Input: part model. Units: mm. Frame: model coordinates. Face numbers are marked on the shaded views. A direction names the side the tool comes from. Coordinates: 2 decimals unless noted, no trailing zeros. Write each loop counter-clockwise with the first axis right and the second up, starting at its lowest first coordinate (ties: lowest second). Pieces come first, ordered by that corner, then holes. Notation, with made-up numbers: M -3,64 L 37,64 A18 cw 37,78 Z; hole C 88,-9 d6. An arc over 180 degrees is marked long. Answer as a JSON object with one key per item and string values. Group by question number.
from build123d import *

# Parameters (mm, degrees)
SKETCH1_W           = 27.94
SKETCH1_H           = 25.4
SKETCH1_W_2         = 25.908
SKETCH1_H_2         = 24.13
BOSS_EXTRUDE1_DEPTH = 2.032
SKETCH2_W           = 27.94
SKETCH2_H           = 25.4
BOSS_EXTRUDE2_DEPTH = 2.54
SKETCH3_R           = 13.843
BOSS_EXTRUDE3_DEPTH = 6.35
FILLET1_R           = 2.54


with BuildPart() as part:
    # Sketch1 → Boss-Extrude1 (new body)
    with BuildSketch(Plane(origin=(0, 0, 0), x_dir=(1, 0, 0), z_dir=(0, 1, 0))):
        Rectangle(SKETCH1_W, SKETCH1_H)
        Rectangle(SKETCH1_W_2, SKETCH1_H_2, mode=Mode.SUBTRACT)
    extrude(amount=BOSS_EXTRUDE1_DEPTH)

    # Sketch2 → Boss-Extrude2 (add)
    with BuildSketch(Plane(origin=(0, 0, 0), x_dir=(1, 0, 0), z_dir=(0, 1, 0))):
        Rectangle(SKETCH2_W, SKETCH2_H)
    extrude(amount=-BOSS_EXTRUDE2_DEPTH)

    # Sketch3 → Boss-Extrude3 (add)
    with BuildSketch(Plane.XZ.offset(2.54)):
        Circle(SKETCH3_R)
    extrude(amount=BOSS_EXTRUDE3_DEPTH)

    # Fillet1
    fillet1_edges = [part.edges().sort_by_distance(p)[0] for p in [
        (13.97, -0.254, 12.7),
        (-13.97, -0.254, 12.7),
        (-13.97, -0.254, -12.7),
        (13.97, -0.254, -12.7),
    ]]
    fillet(fillet1_edges, radius=FILLET1_R)


solid = part.part
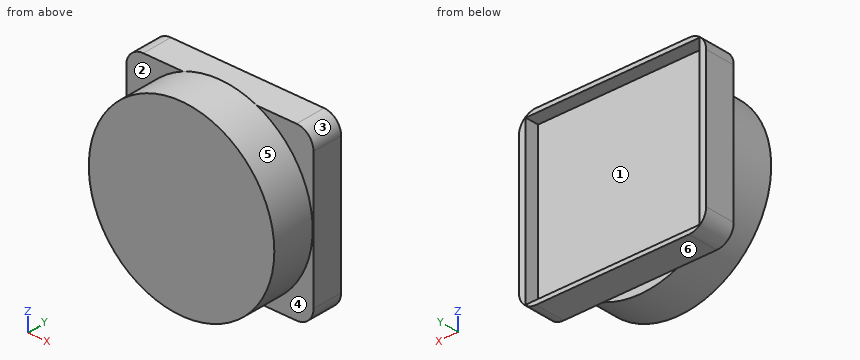
Q1. Access query for the marked faces 4, 5 and 6. Directions: +Z, -Z, +X, -X, +Y, -Y. A direction counts if a zero-diameter tool reaches every point of the face in a straight line with its end or side. Return the directions, or none.
Q2. Draft query along X for the marked faces 1, 2 and 3. Return one class per face: released by +X, released by -X, zero draft, split by the parting line, or undercut.
Q3. Pin query (flat end, axial travel): pin 1 Ø10 at (x, z) = (1.5, 6.5) entering from +Y; pin 2 Ø2.5 at (x, y) = (-2, -1) entering from +Z; pin 3 Ø0.6 at (x, y) = (4, 1.5) entering from -Z. Return the tip coordinate at first contact, or that it passes through.
Q4. Section C-C, the plane x = 0. Return the cut outline in (y, z) (3 decimals), and give its area (3 significant figures).
Q5. Section A-A, the plane y = 0.75. Return the cut outline in (x, z) (3 decimals), and give its area (3 significant figures).
Q6. Section D-D, the plane y = -1.75. Return the cut outline in (x, z).
Q7. Section B-B, the plane z = 0. Return the cut outline in (x, y), and give its area (3 significant figures).
Q8. Line query: line 1 (Z direction, x = -6.75, y = 1) (3 decimals); line 2 (X direction, y = 1.5, z = -5.75); line 3 (Y direction, x = 10.5, z = -1.25). Output: solid intervals per line, ascending. Write a range as from..to.
Filled in:
{
 "1": {"face 4": "+X, -Y", "face 5": "-Y", "face 6": "-Z, +X, -X, +Y"},
 "2": {"face 1": "undercut", "face 2": "zero draft", "face 3": "released by +X"},
 "3": {"pin 1": "y = 0", "pin 2": "z = 12.7", "pin 3": "z = -12.7"},
 "4": {"outline": "M -8.89,-13.843 L -2.54,-13.843 L -2.54,-12.7 L 2.032,-12.7 L 2.032,-12.065 L 0,-12.065 L 0,12.065 L 2.032,12.065 L 2.032,12.7 L -2.54,12.7 L -2.54,13.843 L -8.89,13.843 Z", "area": "243 mm^2"},
 "5": {"outline": "M -13.97,-10.16 A2.54 ccw -11.43,-12.7 L 11.43,-12.7 A2.54 ccw 13.97,-10.16 L 13.97,10.16 A2.54 ccw 11.43,12.7 L -11.43,12.7 A2.54 ccw -13.97,10.16 Z; hole M -12.954,-12.065 L 12.954,-12.065 L 12.954,12.065 L -12.954,12.065 Z", "area": "79.0 mm^2"},
 "6": {"outline": "M -13.97,-10.16 A2.54 ccw -11.43,-12.7 L 11.43,-12.7 A2.54 ccw 13.97,-10.16 L 13.97,10.16 A2.54 ccw 11.43,12.7 L -11.43,12.7 A2.54 ccw -13.97,10.16 Z"},
 "7": {"outline": "M -13.97,-2.54 L -13.84,-2.54 L -13.84,-8.89 L 13.84,-8.89 L 13.84,-2.54 L 13.97,-2.54 L 13.97,2.03 L 12.95,2.03 L 12.95,0 L -12.95,0 L -12.95,2.03 L -13.97,2.03 Z", "area": "251 mm^2"},
 "8": {"line 1": "-12.7..-12.065, 12.065..12.7", "line 2": "-13.97..-12.95, 12.95..13.97", "line 3": "-8.89..0"}
}
